Source: three-view drawing plus pictorial views. Frame: mm from the lowest corner of the part. A direction names the side the tool comes from. Give positions to 0.01 mm unless a question says otherwise; leave off trailing zeros. Loops run counter-clockwise (first coordinate to the right, second up) from the corner with the lowest first, then second, coordinate; pieces in that order, holes last. Notation, with made-up numbers: (61, 37.25) -> (66, 37.25) arc R26 ccw to (66, 64.25) -> close; hole circle Ø11 at (-26, 45). An arc over 180 degrees is marked (long way). Put each result on its own line as item: value.
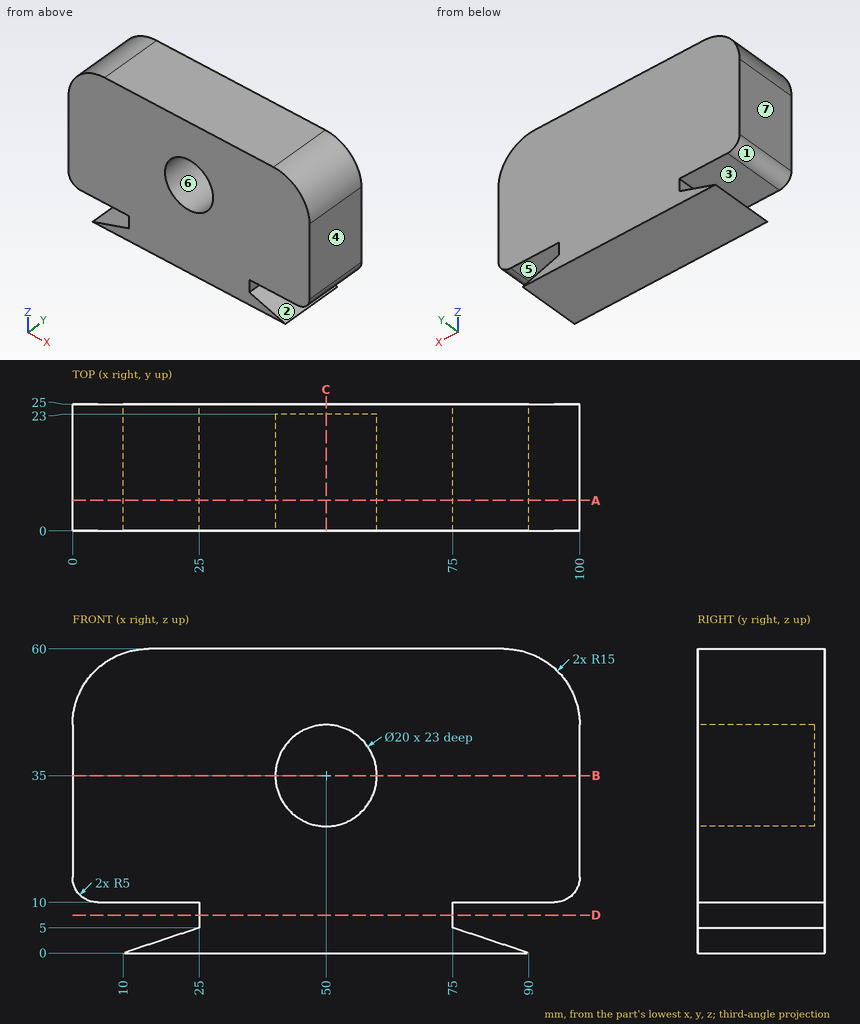
(1) Section A-A on y = 6. Return loops of the section in (x, z).
Calculated:
outline: (0, 15) arc R5 ccw to (5, 10) -> (25, 10) -> (25, 5) -> (10, 0) -> (90, 0) -> (75, 5) -> (75, 10) -> (95, 10) arc R5 ccw to (100, 15) -> (100, 45) arc R15 ccw to (85, 60) -> (15, 60) arc R15 ccw to (0, 45) -> close; hole circle Ø20 at (50, 35)
(2) Section C-C on x = 50. Return loops of the section in (y, z), then the cut area to 3 significant figures.
Calculated:
outline: (0, 0) -> (25, 0) -> (25, 60) -> (0, 60) -> (0, 45) -> (23, 45) -> (23, 25) -> (0, 25) -> close
area: 1,040 mm²
(3) Draft query along X for the marked faces 4, 5, 6 and 7. Return one class per face: released by +X, released by -X, zero draft, split by the parting line, or undercut.
Calculated:
face 4: released by +X
face 5: zero draft
face 6: undercut
face 7: released by -X
(4) Section D-D on z = 7.5. Return loops of the section in (x, y).
Calculated:
outline: (25, 0) -> (75, 0) -> (75, 25) -> (25, 25) -> close
(5) Line query: probe 1 along Z at (x, y) = (50, 16.5); probe 2 along Z at (x, y) = (84, 18.75); probe 3 along X at (y, z) = (14.25, 29). Output: solid intervals per line, ascending. Write a range as from..to.
Calculated:
probe 1: z = 0..25, 45..60
probe 2: z = 0..2, 10..60
probe 3: x = 0..42, 58..100
(6) Reachability of the marked faces 1, 2 and 3 from +Z, -Z, +X, -X, +Y, -Y: full face, straight path, thin tool, end or side. Return the list, or none.
Calculated:
face 1: -Z, -X, +Y, -Y
face 2: +X, +Y, -Y
face 3: -X, +Y, -Y
(7) First-contact query: P1, Ø1.5, axis at y = 13, z = 7.5, coming from the -X side; P2, Ø2.5, axis at y = 14.5, z = 7, coming from the +X side. Flat tips, straight axial feed; report the tip coordinate or a pass-through.
Calculated:
P1: stops at x = 25
P2: stops at x = 75
(8) Section B-B on z = 35. Return loops of the section in (x, y).
Calculated:
outline: (0, 0) -> (40, 0) -> (40, 23) -> (60, 23) -> (60, 0) -> (100, 0) -> (100, 25) -> (0, 25) -> close
